Geometry: final body of the model. Coordinates: model frame, mm. Face numbers are marked on the shaded views. Coordinates: 2 decimals unless noted, no trailing zeros. Write each loop counter-clockwise with the first axis right and the second up, starting at its lowest first coordinate (ties: lowest second). Pieces come first, ordered by that corner, then holes. Notation, with made-up numbers: (-26.75, 24) -> (-9.75, 24) arc R17 cw to (-9.75, 39) -> close; hole circle Ø4 at (27, 39.5). An arc over 180 degrees is marked (long way). One line per item, written item: value.
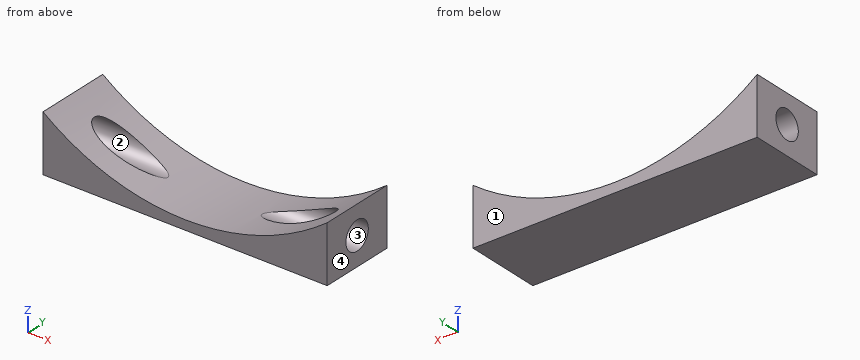
```python
from build123d import *

# Parameters (mm, degrees)
CYLINDER2792_R     = 1.5
CYLINDER2792_DEPTH = 64
CYLINDER2791_R     = 38
CYLINDER2791_DEPTH = 30
BOX975_W           = 2
BOX975_H           = 6
BOX975_DEPTH       = 6
BOX976_W           = 2
BOX976_H           = 6
BOX976_DEPTH       = 6
BOX977_W           = 2
BOX977_H           = 6
BOX977_DEPTH       = 6
BOX978_W           = 2
BOX978_H           = 6
BOX978_DEPTH       = 6
BOX979_W           = 2
BOX979_H           = 6
BOX979_DEPTH       = 6
BOX981_W           = 2
BOX981_H           = 6
BOX981_DEPTH       = 6
TUBE137_R          = 21
TUBE137_R_2        = 2
TUBE137_DEPTH      = 64
TUBE138_R          = 25
TUBE138_R_2        = 2
TUBE138_DEPTH      = 26
BOX980_W           = 30
BOX980_H           = 64
BOX980_DEPTH       = 18
BOX974_W           = 30
BOX974_H           = 8
BOX974_DEPTH       = 18


with BuildPart() as obj1:
    # Cylinder2792 → Cylinder2792 (new body)
    with BuildSketch(Plane(origin=(-26, -13, 14), x_dir=(0, 0, -1), z_dir=(1, 0, 0))):
        Circle(CYLINDER2792_R)
    extrude(amount=CYLINDER2792_DEPTH)


with BuildPart() as obj2:
    # Cylinder2791 → Cylinder2791 (new body)
    with BuildSketch(Plane.XY):
        Circle(CYLINDER2791_R)
    extrude(amount=CYLINDER2791_DEPTH)


with BuildPart() as krychle974:
    # Box975 → Box975 (new body)
    with BuildSketch(Plane(origin=(-12, -4, 10), x_dir=(1, 0, 0), z_dir=(0, 0, 1))):
        with Locations((1, 3)):
            Rectangle(BOX975_W, BOX975_H)
    extrude(amount=BOX975_DEPTH)


with BuildPart() as krychle975:
    # Box976 → Box976 (new body)
    with BuildSketch(Plane(origin=(10, 26, 10), x_dir=(1, 0, 0), z_dir=(0, 0, 1))):
        with Locations((1, 3)):
            Rectangle(BOX976_W, BOX976_H)
    extrude(amount=BOX976_DEPTH)


with BuildPart() as krychle976:
    # Box977 → Box977 (new body)
    with BuildSketch(Plane(origin=(-12, 26, 10), x_dir=(1, 0, 0), z_dir=(0, 0, 1))):
        with Locations((1, 3)):
            Rectangle(BOX977_W, BOX977_H)
    extrude(amount=BOX977_DEPTH)


with BuildPart() as krychle977:
    # Box978 → Box978 (new body)
    with BuildSketch(Plane(origin=(10, 12, 10), x_dir=(1, 0, 0), z_dir=(0, 0, 1))):
        with Locations((1, 3)):
            Rectangle(BOX978_W, BOX978_H)
    extrude(amount=BOX978_DEPTH)


with BuildPart() as krychle978:
    # Box979 → Box979 (new body)
    with BuildSketch(Plane(origin=(-12, 12, 10), x_dir=(1, 0, 0), z_dir=(0, 0, 1))):
        with Locations((1, 3)):
            Rectangle(BOX979_W, BOX979_H)
    extrude(amount=BOX979_DEPTH)


with BuildPart() as compound1243:
    # Box981 → Box981 (new body)
    with BuildSketch(Plane(origin=(10, -4, 10), x_dir=(1, 0, 0), z_dir=(0, 0, 1))):
        with Locations((1, 3)):
            Rectangle(BOX981_W, BOX981_H)
    extrude(amount=BOX981_DEPTH)

    # Compound1243: union Krychle974, Krychle975, Krychle976, Krychle977, Krychle978
    add(krychle974.part)
    add(krychle975.part)
    add(krychle976.part)
    add(krychle977.part)
    add(krychle978.part)


with BuildPart() as tube137:
    # Tube137 → Tube137 (new body)
    with BuildSketch(Plane(origin=(0, 61, 37), x_dir=(1, 0, 0), z_dir=(0, -1, 0))):
        Circle(TUBE137_R)
        Circle(TUBE137_R_2, mode=Mode.SUBTRACT)
    extrude(amount=TUBE137_DEPTH)


with BuildPart() as tube138:
    # Tube138 → Tube138 (new body)
    with BuildSketch(Plane(origin=(0, -3, 37), x_dir=(1, 0, 0), z_dir=(0, -1, 0))):
        Circle(TUBE138_R)
        Circle(TUBE138_R_2, mode=Mode.SUBTRACT)
    extrude(amount=TUBE138_DEPTH)


with BuildPart() as common007:
    # Box980 → Box980 (new body)
    with BuildSketch(Plane(origin=(-15, -17, 11), x_dir=(1, 0, 0), z_dir=(0, 0, 1))):
        with Locations((15, 32)):
            Rectangle(BOX980_W, BOX980_H)
    extrude(amount=BOX980_DEPTH)

    # Cut1049: cut Tube138
    add(tube138.part, mode=Mode.SUBTRACT)

    # Cut1050: cut Tube137
    add(tube137.part, mode=Mode.SUBTRACT)

    # Cut1051: cut Compound1243
    add(compound1243.part, mode=Mode.SUBTRACT)

    # Common007: intersect obj2
    add(obj2.part, mode=Mode.INTERSECT)


with BuildPart() as cut1052:
    # Box974 → Box974 (new body)
    with BuildSketch(Plane(origin=(-15, -17, 11), x_dir=(1, 0, 0), z_dir=(0, 0, 1))):
        with Locations((15, 4)):
            Rectangle(BOX974_W, BOX974_H)
    extrude(amount=BOX974_DEPTH)

    # Common008: intersect Common007
    add(common007.part, mode=Mode.INTERSECT)

    # Cut1052: cut obj1
    add(obj1.part, mode=Mode.SUBTRACT)


solid = cut1052.part
```
(1) Section C-C (x = -13). Return the cut outline in (y, z).
Responses:
outline: (-17, 11) -> (-9, 11) -> (-9, 15.65) -> (-17, 15.65) -> close; hole circle Ø3 at (-13, 14)
(2) Section B-B (y = -13). Return the cut outline in (x, z), then the cut area to 3 significant figures.
Responses:
outline: (-15, 11) -> (15, 11) -> (15, 12.5) -> (4.97, 12.5) arc R25 cw to (-4.97, 12.5) -> (-15, 12.5) -> close; (-15, 15.5) -> (-12.76, 15.5) arc R25 cw to (-15, 17) -> close; (12.76, 15.5) -> (15, 15.5) -> (15, 17) arc R25 cw to start
area: 44.9 mm2
(3) Pull-direction query (Y, two-part tool) for the marked faces 1, 2, 3 and 4; classes: released by +Y, released by -Y, zero draft, split by the parting line, or undercut.
Responses:
face 1: released by +Y
face 2: undercut
face 3: undercut
face 4: zero draft
(4) First-contact query: pin 1 (3 mm diameter, centred on x = -11, y = -16, fed in from +Z); pin 2 (2.5 mm diameter, centred on y = -13, z = 14, fed in from +X). Flat tips, straight axial feed; report the tip coordinate or a pass-through.
Responses:
pin 1: stops at z = 15.35
pin 2: passes through
(5) Section A-A (z = 14). Return the cut outline in (x, y).
Responses:
outline: (-15, -17) -> (-9.8, -17) -> (-9.8, -14.5) -> (-15, -14.5) -> close; (-15, -11.5) -> (-9.8, -11.5) -> (-9.8, -9) -> (-15, -9) -> close; (9.8, -17) -> (15, -17) -> (15, -14.5) -> (9.8, -14.5) -> close; (9.8, -11.5) -> (15, -11.5) -> (15, -9) -> (9.8, -9) -> close
(6) Section D-D (y = -9.75). Return the cut outline in (x, z), then the cut area to 3 significant figures.
Responses:
outline: (-15, 11) -> (15, 11) -> (15, 17) arc R25 cw to (-15, 17) -> close
area: 77.8 mm2
(7) Line query: line 1 (Z direction, x = 10, y = -13); line 2 (Y direction, x = -10.5, z = 14); line 3 (Y direction, x = 11.5, z = 13.25). Output: solid intervals per line, ascending. Write a range as [from, to].
Responses:
line 1: z = [11, 12.5]
line 2: y = [-17, -14.5], [-11.5, -9]
line 3: y = [-17, -14.3], [-11.7, -9]
